Source: CAD feature listing. Evaluate the final solid. Frame: model axes, mm. A direction names the side the tool comes from. Round coordinates to 2 decimals unless told otherwise and drop trailing zeros. Loops run counter-clockwise (first coordinate to the right, second up) from the corner with the lowest first, then second, coordinate; pieces in that order, holes last. Notation, with made-up numbers: (-12.75, -33) - (40.25, -33) arc R34 cw to (40.25, 6) - close; hole circle Ø4 at (-10, 19.5). An arc over 180 degrees is marked (long way). One line per question, with ' | ' between items.
from build123d import *

# Parameters (mm, degrees)
SKETCH_1_W       = 105
SKETCH_1_H       = 67
EXTRUDE_1_DEPTH  = 1
SKETCH_2_W       = 104
SKETCH_2_H       = 66
EXTRUDE_2_DEPTH  = 1
SKETCH_3_W       = 106.5
SKETCH_3_H       = 68.7
EXTRUDE_3_DEPTH  = 3.7
SKETCH_4_W       = 0.4
SKETCH_4_H       = 66
EXTRUDE_4_DEPTH  = 1.5
SKETCH_5_R       = 1.6
EXTRUDE_5_DEPTH  = 0.4
SKETCH_7_W       = 45
SKETCH_7_H       = 38
EXTRUDE_6_DEPTH  = 1.2
SKETCH_8_W       = 7.7
SKETCH_8_H       = 15
EXTRUDE_7_DEPTH  = 5.8
SKETCH_8_3_W     = 8.5
SKETCH_8_3_H     = 8.5
EXTRUDE_8_DEPTH  = 3
SKETCH_8_4_W     = 21
SKETCH_8_4_H     = 4.5
EXTRUDE_9_DEPTH  = 2
SKETCH_8_5_W     = 12
SKETCH_8_5_H     = 15.2
SKETCH_8_5_W_2   = 3
EXTRUDE_10_DEPTH = 2
EXTRUDE_START    = -37.4
EXTRUDE_11_DEPTH = 12.8


with BuildPart() as part:
    # Sketch 1 → Extrude 1 (new body)
    with BuildSketch(Plane(origin=(0, 0, 0), x_dir=(1, 0, 0), z_dir=(0, 1, 0))):
        Rectangle(SKETCH_1_W, SKETCH_1_H)
    extrude(amount=-EXTRUDE_1_DEPTH)

    # Sketch 2 → Extrude 2 (add)
    with BuildSketch(Plane.XZ.offset(1)):
        Rectangle(SKETCH_2_W, SKETCH_2_H)
    extrude(amount=EXTRUDE_2_DEPTH)

    # Sketch 3 → Extrude 3 (add)
    with BuildSketch(Plane.XZ.offset(2)):
        Rectangle(SKETCH_3_W, SKETCH_3_H)
    extrude(amount=EXTRUDE_3_DEPTH)

    # Sketch 4 → Extrude 4 (add)
    with BuildSketch(Plane.XZ.offset(5.7)):
        with Locations((-53.05, 0)):
            Rectangle(SKETCH_4_W, SKETCH_4_H)
        with Locations((53.05, 0)):
            Rectangle(SKETCH_4_W, SKETCH_4_H)
    extrude(amount=EXTRUDE_4_DEPTH)

    # Sketch 5 → Extrude 5 (add)
    # profile 1 of 2: a face of its own
    with BuildSketch(Plane.XZ.offset(7.2)):
        with BuildLine():
            Line((-55.75, 36.8), (-58.5, 36.8))
            ThreePointArc((-58.5, 36.8), (-60.267766953, 36.067766953), (-61, 34.3))
            Line((-61, 34.3), (-61, -34.3))
            ThreePointArc((-61, -34.3), (-60.267766953, -36.067766953), (-58.5, -36.8))
            Line((-58.5, -36.8), (-55.75, -36.8))
            ThreePointArc((-55.75, -36.8), (-53.982233047, -36.067766953), (-53.25, -34.3))
            Line((-53.25, -34.3), (-53.25, 34.3))
            ThreePointArc((-53.25, 34.3), (-53.982233047, 36.067766953), (-55.75, 36.8))
        make_face()
        with Locations(Location((-57.25, 33, 0), (0, 0, 270))):
            Circle(SKETCH_5_R, mode=Mode.SUBTRACT)
        with Locations(Location((-57.25, -33, 0), (0, 0, 90))):
            Circle(SKETCH_5_R, mode=Mode.SUBTRACT)
    # profile 2 of 2: a face of its own
    with BuildSketch(Plane.XZ.offset(7.2)):
        with BuildLine():
            Line((61, 34.3), (61, -34.3))
            ThreePointArc((61, -34.3), (60.267766953, -36.067766953), (58.5, -36.8))
            Line((58.5, -36.8), (55.75, -36.8))
            ThreePointArc((55.75, -36.8), (53.982233047, -36.067766953), (53.25, -34.3))
            Line((53.25, -34.3), (53.25, 34.3))
            ThreePointArc((53.25, 34.3), (53.982233047, 36.067766953), (55.75, 36.8))
            Line((55.75, 36.8), (58.5, 36.8))
            ThreePointArc((58.5, 36.8), (60.267766953, 36.067766953), (61, 34.3))
        make_face()
        with Locations(Location((57.25, -33, 0), (0, 0, 270))):
            Circle(SKETCH_5_R, mode=Mode.SUBTRACT)
        with Locations(Location((57.25, 33, 0), (0, 0, 90))):
            Circle(SKETCH_5_R, mode=Mode.SUBTRACT)
    extrude(amount=-EXTRUDE_5_DEPTH)

    # Sketch 7 → Extrude 6 (add)
    with BuildSketch(Plane.XZ.offset(5.7)):
        with Locations((-3.85, -10.35)):
            Rectangle(SKETCH_7_W, SKETCH_7_H)
    extrude(amount=EXTRUDE_6_DEPTH)

    # Sketch 8 → Extrude 7 (add)
    with BuildSketch(Plane.XZ.offset(6.9)):
        with Locations((-22.5, -20.85)):
            Rectangle(SKETCH_8_W, SKETCH_8_H)
    extrude(amount=EXTRUDE_7_DEPTH)

    # Sketch 8_3 → Extrude 8 (add)
    with BuildSketch(Plane.XZ.offset(6.9)):
        with Locations((-21.6, 3.4)):
            Rectangle(SKETCH_8_3_W, SKETCH_8_3_H)
    extrude(amount=EXTRUDE_8_DEPTH)

    # Sketch 8_4 → Extrude 9 (add)
    with BuildSketch(Plane.XZ.offset(6.9)):
        with Locations((-0.55, 5.9)):
            Rectangle(SKETCH_8_4_W, SKETCH_8_4_H)
    extrude(amount=EXTRUDE_9_DEPTH)

    # Sketch 8_5 → Extrude 10 (add)
    with BuildSketch(Plane.XZ.offset(6.9)):
        with Locations((12.65, -20.55)):
            Rectangle(SKETCH_8_5_W, SKETCH_8_5_H)
        with Locations((20.15, -20.55)):
            Rectangle(SKETCH_8_5_W_2, SKETCH_8_5_H)
    extrude(amount=EXTRUDE_10_DEPTH)

    # Sketch 9 → Extrude 11 (add)
    with BuildSketch(Plane(origin=(53.25, 0, 0), x_dir=(0, 0, -1), z_dir=(1, 0, 0)).offset(EXTRUDE_START)):
        with BuildLine():
            Line((-33.85, -6.3), (-29.85, -6.3))
            Line((-29.85, -6.3), (-29.85, -6.5))
            Line((-29.85, -6.5), (-33.85, -6.5))
            ThreePointArc((-33.85, -6.5), (-34.98137085, -6.03137085), (-35.45, -4.9))
            Line((-35.45, -4.9), (-35.45, -3))
            ThreePointArc((-35.45, -3), (-34.98137085, -1.86862915), (-33.85, -1.4))
            Line((-33.85, -1.4), (-33, -1.4))
            Line((-33, -1.4), (-33, -1.6))
            Line((-33, -1.6), (-33.85, -1.6))
            ThreePointArc((-33.85, -1.6), (-34.839949494, -2.010050506), (-35.25, -3))
            Line((-35.25, -3), (-35.25, -4.9))
            ThreePointArc((-35.25, -4.9), (-34.839949494, -5.889949494), (-33.85, -6.3))
        make_face()
    extrude(amount=-EXTRUDE_11_DEPTH)


solid = part.part
1. Contact query for flat-ended pins moving along their axis: P1, Ø2.5, axis at y = -3.5, z = 14, coming from the -X side; P2, Ø1.1, axis at y = -1.5, z = -5.5, coming from the +X side; P3, Ø2, axis at y = -8, z = 5.5, coming from the -X side; P4, Ø1.5, axis at x = 13, y = -9, coming from the -Z side. Output: stop coordinate, or through.
Worked out:
P1: stops at x = -53.25 | P2: stops at x = 53.25 | P3: stops at x = -61 | P4: stops at z = -28.15
2. Mould query, pull axis Y, two halves, no side actions, for faces 1 (the flat face through (20, -6.9, -20)), 2 (the flat face through (-22, -9.9, 3)), 3 (the cylindrical face through (-57.2, -7, 34.6)). Classes: released by +Y, released by -Y, zero draft, split by the parting line, or undercut.
Worked out:
face 1: undercut | face 2: released by -Y | face 3: zero draft
3. Section query D-D, the plane z = -2. Return loops of the section in (x, y).
Worked out:
outline: (-61, -7.2) - (-52.85, -7.2) - (-52.85, -5.7) - (-26.35, -5.7) - (-26.35, -6.9) - (18.65, -6.9) - (18.65, -5.7) - (52.85, -5.7) - (52.85, -7.2) - (61, -7.2) - (61, -6.8) - (53.25, -6.8) - (53.25, -2) - (52, -2) - (52, -1) - (52.5, -1) - (52.5, 0) - (-52.5, 0) - (-52.5, -1) - (-52, -1) - (-52, -2) - (-53.25, -2) - (-53.25, -6.8) - (-61, -6.8) - close
4. Material intervals for probe 1 along X at (y, z) = (-6.75, 10); probe 2 along Y at (x, z) = (29, -13.5); probe 3 along Y at (x, z) = (18.5, -14), sorted ascending.
Worked out:
probe 1: x = -53.25 to -52.85, 52.85 to 53.25 | probe 2: y = -5.7 to 0 | probe 3: y = -8.9 to 0
5. Section query C-C, the plane x = -35.5. Return loops of the section in (y, z).
Worked out:
outline: (-5.7, -34.35) - (-2, -34.35) - (-2, -33) - (-1, -33) - (-1, -33.5) - (0, -33.5) - (0, 33.5) - (-1, 33.5) - (-1, 33) - (-2, 33) - (-2, 34.35) - (-5.7, 34.35) - close
6. Section query A-A, the plane x = -57.25. Return loops of the section in (y, z), plus the area to 3 significant figures.
Worked out:
outline: (-7.2, -36.8) - (-6.8, -36.8) - (-6.8, -34.6) - (-7.2, -34.6) - close; (-7.2, -31.4) - (-6.8, -31.4) - (-6.8, 31.4) - (-7.2, 31.4) - close; (-7.2, 34.6) - (-6.8, 34.6) - (-6.8, 36.8) - (-7.2, 36.8) - close | area: 26.9 mm2
7. Section query B-B, the plane z = 22. Return loops of the section in (x, y).
Worked out:
outline: (-61, -7.2) - (-52.85, -7.2) - (-52.85, -5.7) - (52.85, -5.7) - (52.85, -7.2) - (61, -7.2) - (61, -6.8) - (53.25, -6.8) - (53.25, -2) - (52, -2) - (52, -1) - (52.5, -1) - (52.5, 0) - (-52.5, 0) - (-52.5, -1) - (-52, -1) - (-52, -2) - (-53.25, -2) - (-53.25, -6.8) - (-61, -6.8) - close
8. Access query for faces 4 (the flat face through (-1, -8.9, 6)), 5 (the flat face through (-57, -6.8, 1)), 6 (the flat face through (53.25, -4, 0)). Directions: +Z, -Z, +X, -X, +Y, -Y. A direction counts if a zero-diameter tool reaches every point of the face in a straight line with its end or side. Return the directions, or none.
Worked out:
face 4: +Z, -Z, +X, -Y | face 5: +Z, -Z, -X, +Y | face 6: +Z, -Z, +X, +Y
